Study the drawing (mm; zero at the part's minimum x, y, z) and answer. A direction names the side the tool comes from. Coordinates: 2 decimals unless noted, no trailing zeros. Order: outer loops, then holes, each group sorted by start corner. A loop starts at its lowest first (then second) coordinate and runs counter-clockwise, first axis right, second up. Notation, with made-up numbers: (55.25, 66) -> (77.25, 66) arc R19 cw to (77.25, 72) -> close; hole circle Ø5 at (76.25, 66.25). An arc over 180 degrees is marked (long way). Answer in a Markdown table with one row per item. Add a question column.
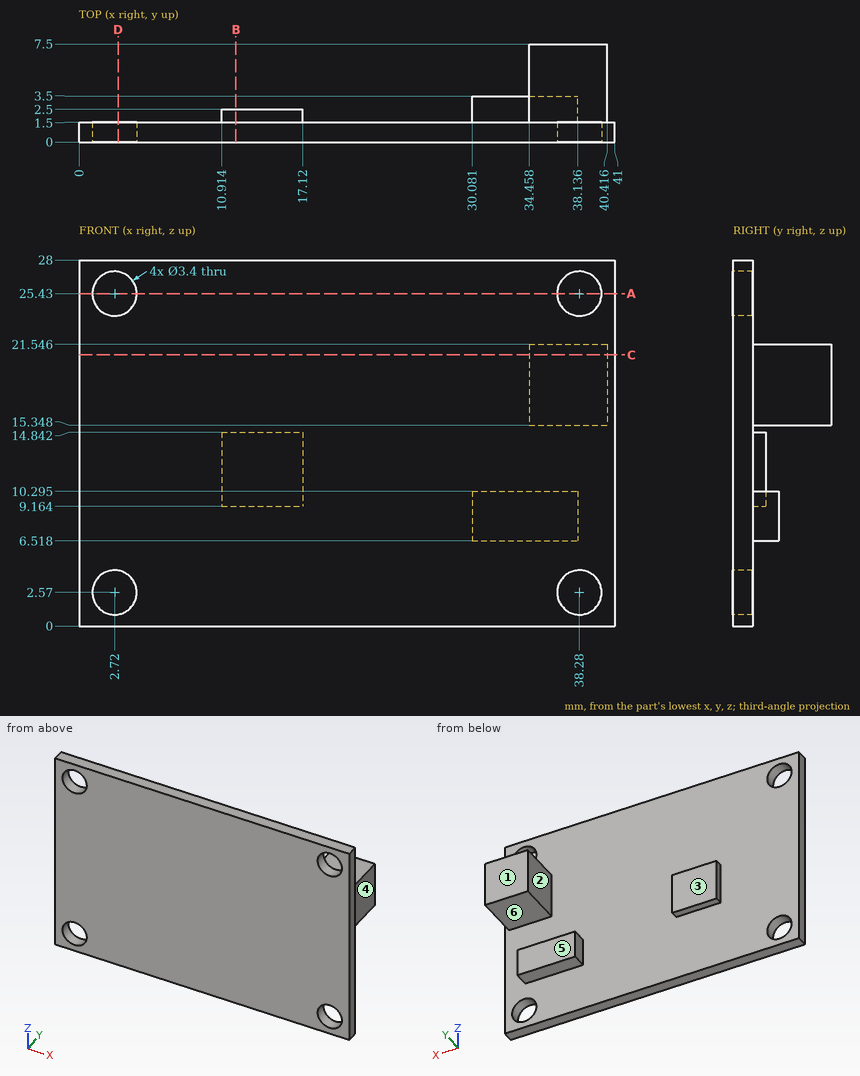
Q1. A cutting plane is placed at C-C (z = 20.75). Determine the outline of the cut face in (x, y).
Q2. For the marked faces 1, 2, 3 and 4, determine the directions among +Z, -Z, +X, -X, +Y, -Y from which every point of the face is accessible in a straight line to the end or side of a thin tool.
Q3. A cutting plane is placed at A-A (z = 25.43). Determine the outline of the cut face in (x, y).
Q4. Straight lines are drawn through the part: line 1 (X direction, y = 0.4, z = 25.43); line 2 (Z direction, x = 38.28, y = 0.6); line 3 (Z direction, x = 38, y = 3.25) (1 decimal). For each, find the intervals that lie inside material, in ascending order.
Q5. A cutting plane is placed at B-B (x = 12). Determine the outline of the cut face in (y, z).
Q6. A cutting plane is placed at D-D (x = 3). Determine the outline of the cut face in (y, z).
Q7. Given pin 1 (6 mm diameter, centred on x = 36, z = 4.5, fed in from +Y); pin 2 (2 mm diameter, centred on y = 3.5, z = 10, fed in from +X); pin 3 (4.5 mm diameter, centred on x = 38.28, z = 2.57, fed in from +Y), each flat-ended and moving along its own axis, determine where each tip first touches the part or whether it passes through.
Q8. Determine the mould class of the marked faces 5 and 6 for opening direction Z: +Z half, -Z half, draft (parallel to the pull), parting line (faces both ways), or undercut.
Returned:
| question | item | result |
|---|---|---|
| 1 | outline | (0, 0) -> (41, 0) -> (41, 1.5) -> (40.42, 1.5) -> (40.42, 7.5) -> (34.46, 7.5) -> (34.46, 1.5) -> (0, 1.5) -> close |
| 2 | face 1 | +Z, -Z, +X, -X, +Y |
| 2 | face 2 | +Z, -X, +Y |
| 2 | face 3 | +Z, -Z, -X, +Y |
| 2 | face 4 | +Z, -Z, +X, +Y |
| 3 | outline | (0, 0) -> (1.02, 0) -> (1.02, 1.5) -> (0, 1.5) -> close; (4.42, 0) -> (36.58, 0) -> (36.58, 1.5) -> (4.42, 1.5) -> close; (39.98, 0) -> (41, 0) -> (41, 1.5) -> (39.98, 1.5) -> close |
| 4 | line 1 | x = 0 to 1.02, 4.42 to 36.58, 39.98 to 41 |
| 4 | line 2 | z = 0 to 0.87, 4.27 to 23.73, 27.13 to 28 |
| 4 | line 3 | z = 6.5 to 10.3, 15.3 to 21.5 |
| 5 | outline | (0, 0) -> (1.5, 0) -> (1.5, 9.16) -> (2.5, 9.16) -> (2.5, 14.84) -> (1.5, 14.84) -> (1.5, 28) -> (0, 28) -> close |
| 6 | outline | (0, 0) -> (1.5, 0) -> (1.5, 0.89) -> (0, 0.89) -> close; (0, 4.25) -> (1.5, 4.25) -> (1.5, 23.75) -> (0, 23.75) -> close; (0, 27.11) -> (1.5, 27.11) -> (1.5, 28) -> (0, 28) -> close |
| 7 | pin 1 | stops at y = 3.5 |
| 7 | pin 2 | stops at x = 38.14 |
| 7 | pin 3 | stops at y = 1.5 |
| 8 | face 5 | draft |
| 8 | face 6 | undercut |
